Could you check a few things on this model? Use its own coordinates, in mm. A direction names the side the tool comes from. Give positions to 0.01 mm unless a question says otherwise; leave off trailing zeros. Loops run counter-clockwise (first coordinate to the right, second up) from the corner with the lowest first, then second, coordinate; pieces in that order, holes last. Notation, with made-up numbers: M 8,13.25 L 27,13.25 A20 cw 27,27.25 Z; hole C 32,3.5 d3. An arc over 180 degrees is marked long. Use a Markdown table: item, result. Add a question column.
1) If I drill on line 1 along Z through (x, y) = (2.5, 1); line 2 along Z through (x, y) = (2.75, -4.25); line 3 along Y through (x, z) = (1.25, 7.5), over which ranges is the centre line in solid material (lowest first)? Write a range as [from, to].
2) We'd pull the mould along Z, two halves only. Please class faces 4 (the conical face through (-2.634, 0.082, 12.365)), 5 (the flat face through (4.75, 0, -4)), 6 (the flat face through (0, 0, -7.4)): +Z half, -Z half, draft (parallel to the pull), parting line (faces both ways), or undercut.
3) Suppose I cut it at C-C on z = 6.5. List the corners of the cut face in (x, y) for me.
4) Which directions (+Z, -Z, +X, -X, +Y, -Y) give clear straight access to the entire face, cutting with the end or side of a thin tool? Please do faces 1 (the flat face through (0, -5.4, -4)), 2 (the cylindrical face through (-2.4, -1.8, 8.5)), 3 (the flat face through (1.5, 0, 9)).
5) Suppose I cut it at B-B on x = 0. List the corners of the cut face in (y, z) for me, and give its area (3 significant figures).
6) Suppose I cut it at A-A on y = 0. List the corners of the cut face in (x, z) for me, and give its area (3 significant figures).
7) Will these pins go through, and if not, where does the flat tip stop? pin 1 Ø3 at (x, z) = (-0.5, 2) entering from +Y; pin 2 Ø1.5 at (y, z) = (-2, 1) entering from +X; pin 3 Ø1.6 at (y, z) = (-0.5, 9) entering from +X.
8) Suppose I cut it at D-D on x = 3.25. List the corners of the cut face in (y, z) for me, and give its area (3 significant figures).
```python
from build123d import *

# Parameters (mm, degrees)
SKETCH_W     = 9.5
SKETCH_H     = 10.8
PAD_DEPTH    = 7.4
SKETCH001_R  = 3.5
PAD001_DEPTH = 5
SKETCH002_R  = 3
PAD002_DEPTH = 12.5
SKETCH003_W  = 1.5
SKETCH003_H  = 7
POCKET_DEPTH = 3
CHAMFER_SIZE = 0.5


with BuildPart() as part:
    # Sketch → Pad (new body)
    with BuildSketch(Plane.XY):
        Rectangle(SKETCH_W, SKETCH_H)
    extrude(amount=-PAD_DEPTH)

    # Sketch001 → Pad001 (join)
    with BuildSketch(Plane.XY):
        Circle(SKETCH001_R)
    extrude(amount=PAD001_DEPTH)

    # Sketch002 → Pad002 (join)
    with BuildSketch(Plane.XY):
        Circle(SKETCH002_R)
    extrude(amount=PAD002_DEPTH)

    # Sketch003 → Pocket (cut, symmetric)
    with BuildSketch(Plane.XZ):
        with Locations((2.25, 9)):
            Rectangle(SKETCH003_W, SKETCH003_H)
    extrude(amount=POCKET_DEPTH, both=True, mode=Mode.SUBTRACT)

    # Chamfer
    chamfer_edges = [part.edges().sort_by_distance(p)[0] for p in [
        (-3, 0, 12.5),
    ]]
    chamfer(chamfer_edges, length=CHAMFER_SIZE)


solid = part.part
```
Answer block:
| question | item | result |
|---|---|---|
| 1 | line 1 | z = [-7.4, 5.5] |
| 1 | line 2 | z = [-7.4, 0] |
| 1 | line 3 | y = [-2.73, 2.73] |
| 2 | face 4 | +Z half |
| 2 | face 5 | draft |
| 2 | face 6 | -Z half |
| 3 | outline | M 1.5,-2.6 L 1.5,2.6 A3 ccw long Z |
| 4 | face 1 | +Z, -Z, +X, -X, -Y |
| 4 | face 2 | +Z |
| 4 | face 3 | +Z, +X, +Y, -Y |
| 5 | outline | M -5.4,-7.4 L 5.4,-7.4 L 5.4,0 L 3.5,0 L 3.5,5 L 3,5 L 3,12 L 2.5,12.5 L -2.5,12.5 L -3,12 L -3,5 L -3.5,5 L -3.5,0 L -5.4,0 Z |
| 5 | area | 160 mm^2 |
| 6 | outline | M -4.75,-7.4 L 4.75,-7.4 L 4.75,0 L 3.5,0 L 3.5,5 L 3,5 L 3,5.5 L 1.5,5.5 L 1.5,12.5 L -2.5,12.5 L -3,12 L -3,5 L -3.5,5 L -3.5,0 L -4.75,0 Z |
| 6 | area | 140 mm^2 |
| 7 | pin 1 | stops at y = 3.5 |
| 7 | pin 2 | stops at x = 3.27 |
| 7 | pin 3 | stops at x = 1.5 |
| 8 | outline | M -5.4,-7.4 L 5.4,-7.4 L 5.4,0 L 1.3,0 L 1.3,5 L -1.3,5 L -1.3,0 L -5.4,0 Z |
| 8 | area | 92.9 mm^2 |
